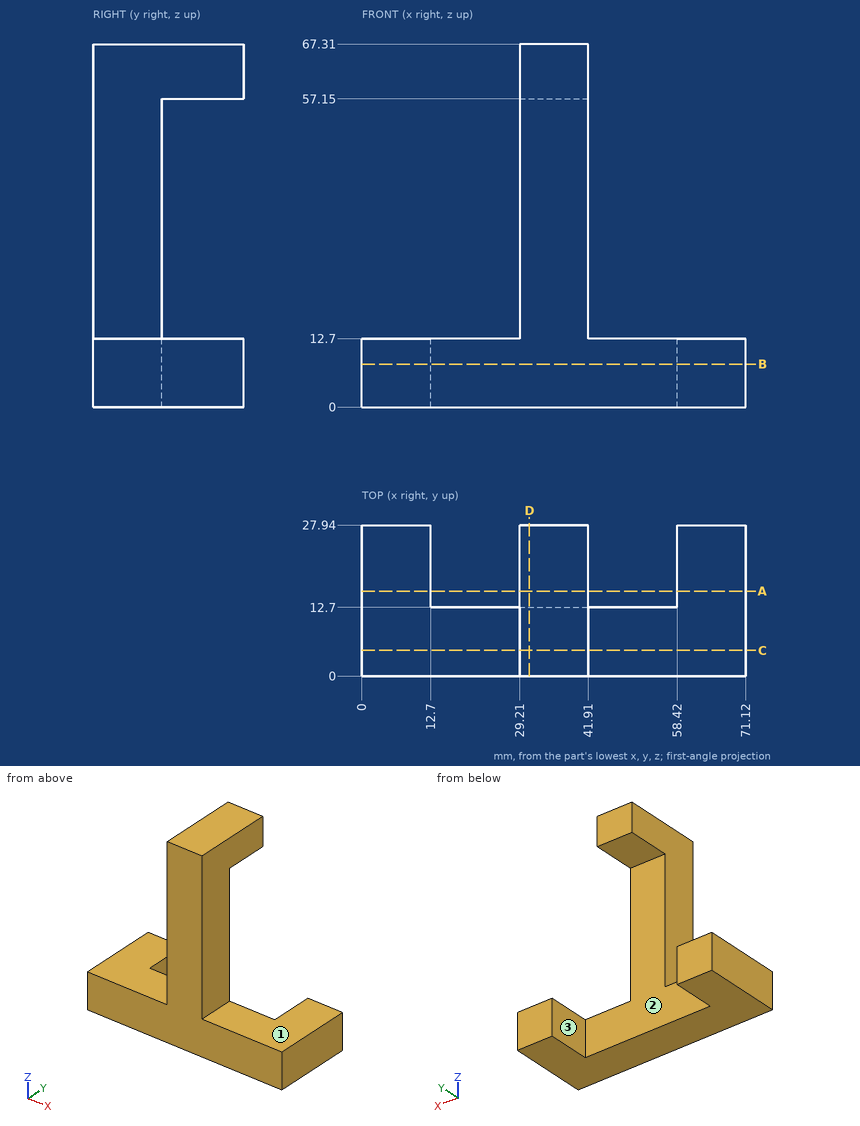
Study the drawing (mm; zero at the part's minimum x, y, z) and answer. A direction names the side the tool comes from. Round coordinates to 2 decimals unless told otherwise and drop trailing zeros. Write each loop counter-clockwise with the first axis right and the second up, starting at its lowest first coordinate (ties: lowest second). Pieces come first, ordered by that corner, then holes. Notation, with made-up numbers: (2.5, 42.5) - (34.5, 42.5) arc R21 ccw to (34.5, 47.5) - close; hole circle Ø1 at (75, 63). An arc over 180 degrees is marked (long way). Return JSON: item names as keys, results as strings. Group by question number.
Q1. The part is cut by section B-B on z = 8. Write down the section's boundary in (x, y), then the cut area to 3 significant figures.
Q2. The part is cut by section C-C on y = 4.75. Write down the section's boundary in (x, z), then the cut area to 3 significant figures.
Q3. The part is cut by section A-A on y = 15.75. Write down the section's boundary in (x, z).
Q4. For the marked faces 1, 2 and 3, determine the directions among +Z, -Z, +X, -X, +Y, -Y from which every point of the face is accessible in a straight line to the end or side of a thin tool.
Q5. The part is cut by section D-D on x = 31. Write down the section's boundary in (y, z).
Q6. Find the intervals of material crossed by L1, parallel to X at y = 6, z = 35; L2, parallel to Z at x = 56, y = 11.25, in increasing order.
Q7. Each of these flat-tipped pins is pushed along its axis until it touches: pin 1 Ø3 at (y, z) = (3, 27.5) entering from +X; pin 2 Ø8 at (x, y) = (34.5, 25) entering from -Z; pin 3 Ø5 at (y, z) = (4.5, 43.5) entering from -X; pin 4 Ø8 at (x, y) = (22.5, 22) entering from +Z. Where does it stop, or does it pass through?
Solved:
{
 "1": {"outline": "(0, 0) - (71.12, 0) - (71.12, 27.94) - (58.42, 27.94) - (58.42, 12.7) - (12.7, 12.7) - (12.7, 27.94) - (0, 27.94) - close", "area": "1,290 mm²"},
 "2": {"outline": "(0, 0) - (71.12, 0) - (71.12, 12.7) - (41.91, 12.7) - (41.91, 67.31) - (29.21, 67.31) - (29.21, 12.7) - (0, 12.7) - close", "area": "1,600 mm²"},
 "3": {"outline": "(0, 0) - (12.7, 0) - (12.7, 12.7) - (0, 12.7) - close; (29.21, 57.15) - (41.91, 57.15) - (41.91, 67.31) - (29.21, 67.31) - close; (58.42, 0) - (71.12, 0) - (71.12, 12.7) - (58.42, 12.7) - close"},
 "4": {"face 1": "+Z, +X, +Y, -Y", "face 2": "-Z, +Y", "face 3": "+Z, -Z, +Y"},
 "5": {"outline": "(0, 0) - (12.7, 0) - (12.7, 57.15) - (27.94, 57.15) - (27.94, 67.31) - (0, 67.31) - close"},
 "6": {"L1": "29.21 to 41.91", "L2": "0 to 12.7"},
 "7": {"pin 1": "x = 41.91", "pin 2": "z = 57.15", "pin 3": "x = 29.21", "pin 4": "through"}
}
